from build123d import *

# Parameters (mm, degrees)
SM_BASE_FLANGE_1_DEPTH = 50
SKETCH_6_R             = 6.5
CUT_EXTRUDE_1_DEPTH    = 10
SKETCH_7_R             = 6.5
CUT_EXTRUDE_2_DEPTH    = 10
OTHER_START            = 160.088975261
OTHER_1_OUTLINE_W      = 10
OTHER_1_OUTLINE_H      = 8
OTHER_1_DEPTH          = 3.535533906
OTHER_START_2          = 195.44431432
OTHER_1_2_OUTLINE_W    = 39
OTHER_1_2_OUTLINE_H    = 8
OTHER_1_2_DEPTH        = 3.535533906
OTHER_1_3_OUTLINE_W    = 7
OTHER_1_3_OUTLINE_H    = 10
OTHER_1_3_DEPTH        = 3.535533906
OTHER_START_3          = -35.355339059
OTHER_1_4_OUTLINE_W    = 7
OTHER_1_4_OUTLINE_H    = 38
OTHER_1_4_DEPTH        = 3.535533906


# Read off the part's stored shape, not the designer's step: Затупленный угол1
# Sheet-metal steps are written as plain solids
with BuildPart() as part:
    # Sketch 1 → Базовая кромка1 (new body)
    with BuildSketch(Plane.XY):
        with BuildLine():
            Line((231.4, 404.5), (181.4, 404.5))
            ThreePointArc((181.4, 404.5), (174.328932188, 401.571067812), (171.4, 394.5))
            Line((171.4, 394.5), (171.4, 355.894452277))
            ThreePointArc((171.4, 355.894452277), (170.198513935, 350.012189687), (166.786531576, 345.072254634))
            Line((166.786531576, 345.072254634), (3.075645616, 187.951830244))
            ThreePointArc((3.075645616, 187.951830244), (0.80099071, 184.658540209), (0, 180.737031815))
            Line((0, 180.737031815), (0, 0))
            Line((0, 0), (-5, 0))
            Line((-5, 0), (-5, 180.737031815))
            ThreePointArc((-5, 180.737031815), (-3.798513935, 186.619294405), (-0.386531576, 191.559229458))
            Line((-0.386531576, 191.559229458), (163.324354384, 348.679653848))
            ThreePointArc((163.324354384, 348.679653848), (165.59900929, 351.972943883), (166.4, 355.894452277))
            Line((166.4, 355.894452277), (166.4, 394.5))
            ThreePointArc((166.4, 394.5), (170.793398282, 405.106601718), (181.4, 409.5))
            Line((181.4, 409.5), (231.4, 409.5))
            Line((231.4, 409.5), (231.4, 404.5))
        make_face()
    extrude(amount=SM_BASE_FLANGE_1_DEPTH)

    # Эскиз6 → Вырез-Вытянуть1 (cut)
    with BuildSketch(Plane.ZY.offset(5)):
        with Locations(Location((15, 15, 0), (0, 0, 270))):
            Circle(SKETCH_6_R)
        with Locations(Location((15, 40, 0), (0, 0, 270))):
            Circle(SKETCH_6_R)
    extrude(amount=-CUT_EXTRUDE_1_DEPTH, mode=Mode.SUBTRACT)

    # Эскиз7 → Вырез-Вытянуть2 (cut)
    with BuildSketch(Plane(origin=(0, 409.5, 0), x_dir=(1, 0, 0), z_dir=(0, 1, 0))):
        with Locations(Location((206.4, -25, 0), (0, 0, 180))):
            Circle(SKETCH_7_R)
    extrude(amount=-CUT_EXTRUDE_2_DEPTH, mode=Mode.SUBTRACT)

    # Other 1 outline → Other 1 (cut)
    with BuildSketch(Plane(origin=(0, 0, 0), x_dir=(0.707106781186548, 0, 0.707106781186547), z_dir=(0.707106781186547, 0, -0.707106781186548)).offset(OTHER_START)):
        with Locations((164, -407)):
            Rectangle(OTHER_1_OUTLINE_W, OTHER_1_OUTLINE_H)
    extrude(amount=OTHER_1_DEPTH, mode=Mode.SUBTRACT)

    # Other 1 2 outline → Other 1 2 (cut)
    with BuildSketch(Plane(origin=(0, 0, 0), x_dir=(0.707106781186548, 0, -0.707106781186547), z_dir=(0.707106781186547, 0, 0.707106781186548)).offset(OTHER_START_2)):
        with Locations((142.5, 407)):
            Rectangle(OTHER_1_2_OUTLINE_W, OTHER_1_2_OUTLINE_H)
    extrude(amount=OTHER_1_2_DEPTH, mode=Mode.SUBTRACT)

    # Other 1 3 outline → Other 1 3 (cut)
    with BuildSketch(Plane(origin=(0, 0, 0), x_dir=(1, 0, 0), z_dir=(0, 0.707106781186547, 0.707106781186548))):
        with Locations((-2.5, 0)):
            Rectangle(OTHER_1_3_OUTLINE_W, OTHER_1_3_OUTLINE_H)
    extrude(amount=OTHER_1_3_DEPTH, mode=Mode.SUBTRACT)

    # Other 1 4 outline → Other 1 4 (cut)
    with BuildSketch(Plane(origin=(0, 0, 0), x_dir=(1, 0, 0), z_dir=(0, 0.707106781186547, -0.707106781186548)).offset(OTHER_START_3)):
        with Locations((-2.5, -21)):
            Rectangle(OTHER_1_4_OUTLINE_W, OTHER_1_4_OUTLINE_H)
    extrude(amount=OTHER_1_4_DEPTH, mode=Mode.SUBTRACT)


solid = part.part
Could you check a few things on this model? Use its own coordinates, in mm. A direction names the side the tool comes from. Coordinates: 2 decimals unless noted, no trailing zeros. Write each loop counter-clockwise with the first axis right and the second up, starting at its lowest first coordinate (ties: lowest second). Pieces come first, ordered by that corner, then holes. Notation, with made-up numbers: (-25.75, 34) - (13.25, 34) arc R14 cw to (13.25, 50) - close; hole circle Ø8 at (-37.5, -12.75). An arc over 180 degrees is marked (long way). Put each result on its own line as item: value. Start each with the question number.
Q1. Please list where these lines run through material, in increasing order: L1, parallel to Z at x = -2.9, y = 40; L2, parallel to Z at x = 206, y = 406; L3, parallel to X at y = 42, z = 35.5.
Q2. Thinking about a two-plate mould opening in Z: for faces 1 (the cylindrical face through (-2.535, 46.494, 15.286)), 2 (the flat face through (171.4, 375, 25)), 3 (the flat face through (34, 223, 50)), which applies, pulls with the +Z half, pulls with the -Z half, needs draft (parallel to the pull), parting line crosses it, or undercut?
Q3. I want a section at D-D on y = 260.5. Write out the boundary of the cut face in (x, z).
Q4. I'm going to push flat-ended pins straight in: P1, Ø19.5, axis at y = 382.5, z = 19.5, coming from the +X side; P2, Ø10, axis at x = 133, z = 28.5, coming from the -Y side; P3, Ø15, axis at x = 202, z = 20, coming from the -Y side. Where does each tip first touch, or does it pass through?
Q5. I want a section at A-A on y = 15. Write out the boundary of the cut face in (x, z).
Q6. I want a section at B-B on x = 206.4. Write out the boundary of the cut face in (y, z), plus the area to 3 significant figures.
Q7. I want a section at C-C on z = 40. Write out the boundary of the cut face in (x, y), plus the area to 3 significant figures.
Q8. Which directions (+Z, -Z, +X, -X, +Y, -Y) give clear straight access to the entire face, cutting with the end or side of a thin tool? Please do faces 4 (the flat face through (0, 92, 25)), 5 (the flat face through (166.4, 375, 25)), 6 (the cylindrical face through (200.2, 407.04, 26.95)).
Checks:
1. L1: 0 to 8.5, 21.5 to 50
1. L2: 0 to 18.51, 31.49 to 50
1. L3: -5 to 0
2. face 1: undercut
2. face 2: needs draft
2. face 3: pulls with the +Z half
3. outline: (71.45, 0) - (78.67, 0) - (78.67, 50) - (71.45, 50) - close
4. P1: x = 171.4
4. P2: y = 307.85
4. P3: y = 404.5
5. outline: (-5, 0) - (0, 0) - (0, 8.5) - (-5, 8.5) - close; (-5, 21.5) - (0, 21.5) - (0, 50) - (-5, 50) - close
6. outline: (404.5, 0) - (409.5, 0) - (409.5, 18.5) - (404.5, 18.5) - close; (404.5, 31.5) - (409.5, 31.5) - (409.5, 50) - (404.5, 50) - close
6. area: 185 mm²
7. outline: (-5, 0) - (0, 0) - (0, 180.74) arc R10 cw to (3.08, 187.95) - (166.79, 345.07) arc R15 ccw to (171.4, 355.89) - (171.4, 394.5) arc R10 cw to (181.4, 404.5) - (231.4, 404.5) - (231.4, 409.5) - (181.4, 409.5) arc R15 ccw to (166.4, 394.5) - (166.4, 355.89) arc R10 cw to (163.32, 348.68) - (-0.39, 191.56) arc R15 ccw to (-5, 180.74) - close
7. area: 2,680 mm²
8. face 4: +Z, -Z, +X, -Y
8. face 5: +Z, -Z, -X, +Y
8. face 6: +Y, -Y
